Input: part model. Units: mm. Frame: model coordinates. A direction names the side the tool comes from. Round coordinates to 2 decimals unless told otherwise and drop trailing zeros. Order: outer loops, then holes, each group sorted by start corner. A loop starts at its lowest first (then second) coordinate and runs counter-clockwise, first axis right, second up.
Item 1: Cut plane A-A on y = 2.75. Output: boundary loops of the cut face in (x, z), then the cut area to 3 significant figures.
Item 2: Cut plane C-C on x = 39.5. Output: boundary loops of the cut face in (y, z).
Item 3: Line query: L1, parallel to Z at x = 120, y = 4; L2, parallel to X at y = 0.75, z = -30.5; L3, parallel to X at y = 1, z = -89. Output: solid intervals per line, ascending.
Item 4: Reachability of faces 1 (the flat face through (150, 3, -78)), 2 (the flat face through (86, 3, -87)), 3 (the flat face through (150, 3, -33)) from +Z, -Z, +X, -X, +Y, -Y: full face, straight path, thin tool, end or side. Return the list, or none.
Item 5: Cut plane B-B on z = -41. Output: boundary loops of the cut face in (x, y).
Item 6: First-contact query: pin 1 (5 mm diameter, centred on x = 28.5, z = -48, fed in from -Y); pin 2 (3 mm diameter, centred on y = 3, z = -80, fed in from +X); pin 3 (1.9 mm diameter, centred on y = 3, z = -80, fed in from -X). Flat tips, straight axial feed; report the tip coordinate or a pass-through.
Item 7: Mould query, pull axis X, two halves, no side actions, for faces 4 (the flat face through (130.69, 3.13, -90.94)), 5 (the flat face through (137, 3, -95)), 6 (the flat face through (39.31, 3.13, -90.94)), 7 (the cylindrical face through (23.01, 3.13, -22.85)). Classes: released by +X, released by -X, zero draft, split by the parting line, or undercut.
Autodesk Fusion 360 part; units mm, degrees
sketch "Sketch1" plane through (0, 0, 0) normal (0, 1, 0) x (1, 0, 0)
  line L0 (0, 0) -> (170, 0)
  line L1 (170, 0) -> (170, 170)
  line L2 (170, 170) -> (0, 170)
  line L3 (0, 170) -> (0, 0)
  line L4 (85, 170) -> (85, 128.5) construction
  line L5 (110, 107) -> (60, 107)
  line L6 (50, 117) -> (50, 140)
  line L7 (60, 150) -> (110, 150)
  line L8 (120, 140) -> (120, 117)
  line L9 (120, 107) -> (50, 150) construction
  line L10 (50, 107) -> (120, 150) construction
  arc A0 (60, 150) -> (50, 140) centre (60, 140) ccw
  arc A1 (120, 140) -> (110, 150) centre (110, 140) ccw
  arc A2 (110, 107) -> (120, 117) centre (110, 117) ccw
  arc A3 (50, 117) -> (60, 107) centre (60, 117) ccw
  line L11 (85, 128.5) -> (0, 128.5) construction
  line L12 (85, 128.5) -> (170, 128.5) construction
  arc A4 (0, 108.5) -> (0, 148.5) centre (0, 128.5) ccw
  arc A5 (170, 148.5) -> (170, 108.5) centre (170, 128.5) ccw
  line L13 (85, 0) -> (85, 53.5) construction
  line L14 (140, 20) -> (30, 20)
  line L15 (20, 30) -> (20, 87)
  line L16 (150, 87) -> (150, 30)
  line L17 (150, 20) -> (20, 87) construction
  line L18 (20, 20) -> (150, 87) construction
  arc A6 (20, 30) -> (30, 20) centre (30, 30) ccw
  arc A7 (140, 20) -> (150, 30) centre (140, 30) ccw
  line L19 (85, 53.5) -> (20, 53.5) construction
  line L20 (85, 53.5) -> (150, 53.5) construction
  line L21 (20, 53.5) -> (13.5, 53.5) construction
  line L22 (13.5, 53.5) -> (13.5, 64)
  line L23 (13.5, 53.5) -> (13.5, 43)
  line L24 (13.5, 43) -> (13.5, 36.5) construction
  line L25 (13.5, 36.5) -> (20, 36.5) construction
  line L26 (13.5, 64) -> (13.5, 70.5) construction
  line L27 (13.5, 70.5) -> (20, 70.5) construction
  line L28 (13.5, 64) -> (20, 70.5)
  line L29 (13.5, 43) -> (20, 36.5)
  line L30 (156.5, 64) -> (150, 70.5)
  line L31 (156.5, 53.5) -> (156.5, 64)
  line L32 (156.5, 53.5) -> (156.5, 43)
  line L33 (156.5, 43) -> (150, 36.5)
  line L34 (85, 53.5) -> (85, 87) construction
  line L35 (85, 128.5) -> (85, 87) construction
  line L36 (85, 87) -> (43.25, 87)
  line L37 (43.25, 87) -> (35.25, 95)
  line L38 (30, 95) -> (35.25, 95)
  line L39 (35.25, 95) -> (35.25, 87) construction
  line L40 (35.25, 87) -> (43.25, 87) construction
  line L41 (30, 95) -> (30, 85) construction
  arc A8 (30, 95) -> (20, 85) centre (30, 85) ccw
  line L42 (30, 85) -> (30, 95) construction
  line L43 (30, 85) -> (20, 85) construction
  arc A9 (150, 85) -> (140, 95) centre (140, 85) ccw
  line L44 (140, 95) -> (134.75, 95)
  line L45 (126.75, 87) -> (134.75, 95)
  line L46 (85, 87) -> (126.75, 87)
  point P0 (85, 128.5)
  point P1 (85, 53.5)
  dimension "d1" = 170
  dimension "d2" = 170
  dimension "d19" = 41.5
  dimension "d20" = 70
  dimension "d21" = 43
  dimension "d22" = 10
  dimension "d23" = 10
  dimension "d24" = 10
  dimension "d25" = 10
  dimension "d26" = 20
  dimension "d27" = 20
  dimension "d28" = 53.5
  dimension "d29" = 130
  dimension "d30" = 67
  dimension "d31" = 10
  dimension "d32" = 10
  dimension "d33" = 6.5
  dimension "d34" = 10.5
  dimension "d35" = 10.5
  dimension "d36" = 6.5
  dimension "d37" = 6.5
  dimension "d41" = 41.5
  dimension "d42" = 33.5
  dimension "d44" = 41.75
  dimension "d48" = 5.25
  dimension "d49" = 135
  dimension "d50" = 8
  dimension "d51" = 10
  dimension "d52" = 90
  dimension "d53" = 135
  dimension "d54" = 8
extrude "Extrude1" add sketch "Sketch1" along normal blind 6.35 contours L14 L15 L16 A6 A7 L36 L37 L38 A8 A9 L44 L45 L46 | L16 L30 L31 L32 L33 | L15 L22 L23 L28 L29
From the geometry:
1. outline: (13.5, -64) - (20, -70.5) - (20, -85) arc R10 ccw to (30, -95) - (35.25, -95) - (43.25, -87) - (126.75, -87) - (134.75, -95) - (140, -95) arc R10 ccw to (150, -85) - (150, -70.5) - (156.5, -64) - (156.5, -43) - (150, -36.5) - (150, -30) arc R10 ccw to (140, -20) - (30, -20) arc R10 ccw to (20, -30) - (20, -36.5) - (13.5, -43) - close
1. area: 9,290 mm2
2. outline: (0, -90.75) - (6.35, -90.75) - (6.35, -20) - (0, -20) - close
3. L1: z = -87 to -20
3. L2: x = 20 to 150
3. L3: x = 20.83 to 41.25, 128.75 to 149.17
4. face 1: -Z, +X, +Y, -Y
4. face 2: -Z, +Y, -Y
4. face 3: +Z, +X, +Y, -Y
5. outline: (15.5, 0) - (154.5, 0) - (154.5, 6.35) - (15.5, 6.35) - close
6. pin 1: stops at y = 0
6. pin 2: stops at x = 150
6. pin 3: stops at x = 20
7. face 4: undercut
7. face 5: zero draft
7. face 6: undercut
7. face 7: released by -X
